Design review of the part shown in the three views and the two pictorial views. Dimensions are in mm from the part's minimum x, y and z. Coordinates: 2 decimals unless noted, no trailing zeros. Loops run counter-clockwise (first coordinate to the right, second up) from the corner with the lowest first, then second, coordinate; pieces in that order, holes last. Notation, with made-up numbers: (-23, 16.5) -> (3, 16.5) arc R17 ccw to (3, 31.5) -> close; hole circle Ø10 at (-39.75, 44.25). An arc over 180 degrees is marked (long way). Answer in a Markdown table with one row per item.
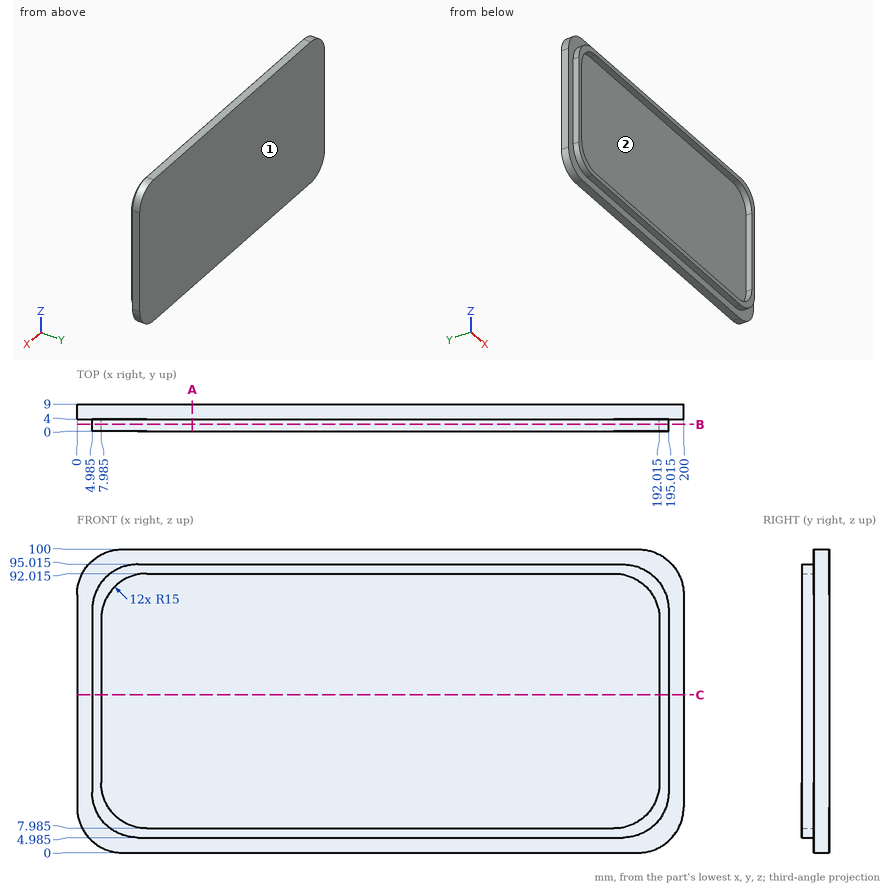
(1) Draft analysis for pull direction X (two halves, no side actions). For the marked faces 1 and 2, state which applies: pulls with the +X half, pulls with the -X half, needs draft (parallel to the pull), parting line crosses it, or undercut.
Evaluation:
| item | result |
|---|---|
| face 1 | needs draft |
| face 2 | undercut |
(2) Take a section at C-C on z = 52. Give the boundary of the cut face in (x, y) (3 decimals).
Evaluation:
| item | result |
|---|---|
| outline | (0, 4) -> (4.985, 4) -> (4.985, 0) -> (7.985, 0) -> (7.985, 4) -> (192.015, 4) -> (192.015, 0) -> (195.015, 0) -> (195.015, 4) -> (200, 4) -> (200, 9) -> (0, 9) -> close |
(3) Take a section at A-A on x = 38. Give the boundary of the cut face in (y, z) (3 decimals), and give its area (3 significant figures).
Evaluation:
| item | result |
|---|---|
| outline | (0, 4.985) -> (4, 4.985) -> (4, 0) -> (9, 0) -> (9, 100) -> (4, 100) -> (4, 95.015) -> (0, 95.015) -> (0, 92.015) -> (4, 92.015) -> (4, 7.985) -> (0, 7.985) -> close |
| area | 524 mm² |
(4) To check wall thickness, follow probe 1 along X at (y, z) = (1, 40) (3 decimals); probe 2 along Z at (x, y) = (172, 2) (3 decimals); probe 3 along Y at (x, z) = (91.5, 26.5). State the ranges of each line that lie inside material, in increasing order.
Evaluation:
| item | result |
|---|---|
| probe 1 | x = 4.985 to 7.985, 192.015 to 195.015 |
| probe 2 | z = 4.985 to 7.985, 92.015 to 95.015 |
| probe 3 | y = 4 to 9 |
(5) For pin 1 (1.2 mm diameter, centred on x = 82, y = 3, fed in from -Z) (3 decimals); pin 2 (1.5 mm diameter, centred on y = 1.5, z = 55.5, fed in from -X) (3 decimals); pin 3 (2 mm diameter, centred on y = 2.5, z = 37, fed in from +X) (3 decimals); pin 4 (1 mm diameter, centred on y = 4.5, z = 77, fed in from -X), all flat-tipped, find the tip position at first contact; note any pin that passes through.
Evaluation:
| item | result |
|---|---|
| pin 1 | stops at z = 4.985 |
| pin 2 | stops at x = 4.985 |
| pin 3 | stops at x = 195.015 |
| pin 4 | stops at x = 0 |
(6) Take a section at B-B on y = 2.25. Give the boundary of the cut face in (x, z) (3 decimals).
Evaluation:
| item | result |
|---|---|
| outline | (4.985, 19.985) arc R15 ccw to (19.985, 4.985) -> (180.015, 4.985) arc R15 ccw to (195.015, 19.985) -> (195.015, 80.015) arc R15 ccw to (180.015, 95.015) -> (19.985, 95.015) arc R15 ccw to (4.985, 80.015) -> close; hole (7.985, 22.985) arc R15 ccw to (22.985, 7.985) -> (177.015, 7.985) arc R15 ccw to (192.015, 22.985) -> (192.015, 77.015) arc R15 ccw to (177.015, 92.015) -> (22.985, 92.015) arc R15 ccw to (7.985, 77.015) -> close |
